Part print with two shaded views. Sizes in mm from the minimum x, y, z corner. Round coordinates to 2 decimals unless told otherwise and drop trailing zeros. Write each loop counter-clockwise with the first axis right and the second up, starting at its lowest first coordinate (ties: lowest second). Pieces come first, ordered by that corner, then holes. Notation, with made-up numbers: (32, 27.25) -> (48, 27.25) arc R23 ccw to (48, 48.25) -> close; hole circle Ø9 at (55.5, -20). An arc over 180 degrees is marked (long way). Return JSON: item names as keys, results as strings.
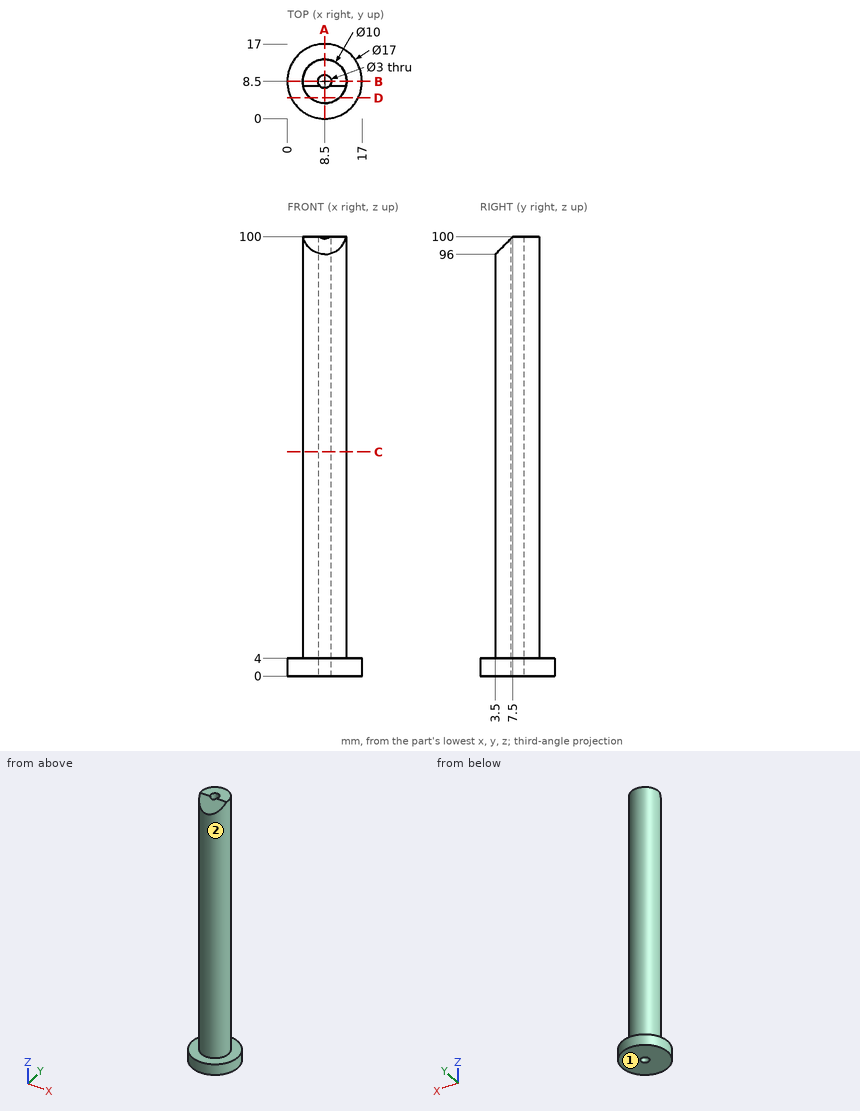
Q1. Saw through at B-B on y = 8.5. List the corners of the cut face in (x, z).
Verdict:
{"outline": "(0, 0) -> (7, 0) -> (7, 100) -> (3.5, 100) -> (3.5, 4) -> (0, 4) -> close; (10, 0) -> (17, 0) -> (17, 4) -> (13.5, 4) -> (13.5, 100) -> (10, 100) -> close"}
Q2. Saw through at D-D on y = 4.75. List the corners of the cut face in (x, z), then the cut area to 3 significant figures.
Verdict:
{"outline": "(0.87, 0) -> (16.13, 0) -> (16.13, 4) -> (11.81, 4) -> (11.81, 97.25) -> (5.19, 97.25) -> (5.19, 4) -> (0.87, 4) -> close", "area": "678 mm²"}
Q3. Saw through at C-C on z = 51. List the corners of the cut face in (x, y), then the cut area to 3 significant figures.
Verdict:
{"outline": "circle Ø10 at (8.5, 8.5); hole circle Ø3 at (8.5, 8.5)", "area": "71.5 mm²"}
Q4. Saw through at A-A on x = 8.5. List the corners of the cut face in (y, z).
Verdict:
{"outline": "(0, 0) -> (7, 0) -> (7, 99.5) -> (3.5, 96) -> (3.5, 4) -> (0, 4) -> close; (10, 0) -> (17, 0) -> (17, 4) -> (13.5, 4) -> (13.5, 100) -> (10, 100) -> close"}
Q5. Two-plate mould, pull along X, no slides. Class the marked faces 1 and 2: +X half, -X half, draft (parallel to the pull), parting line (faces both ways), or undercut.
Verdict:
{"face 1": "draft", "face 2": "parting line"}
Q6. Pin check, flat tips, straight feed: pin 1 Ø1 at (x, z) = (6, 35.5) entering from +Y; pin 2 Ø2 at (y, z) = (12, 58) entering from +X; pin 3 Ø6 at (x, z) = (3.5, 61.5) entering from -Y; pin 4 Ø1.8 at (x, y) = (8.5, 8.5) entering from -Z. Stop position of each tip, or through.
Verdict:
{"pin 1": "stops at y = 13.08", "pin 2": "stops at x = 12.83", "pin 3": "stops at y = 3.92", "pin 4": "passes through"}
Q7. Wall check: L1, parallel to X at y = 8.5, z = 58; L2, parallel to Z at x = 1.5, y = 5.75. Give the ranges that are in metal, low to high.
Verdict:
{"L1": "x = 3.5 to 7, 10 to 13.5", "L2": "z = 0 to 4"}
